Build history of the part. All positions in model axes, mm. A direction names the side the tool comes from. Round coordinates to 2 decimals unless told otherwise and drop trailing zeros. Write each loop counter-clockwise with the first axis right and the second up, starting at its lowest first coordinate (ties: lowest second). Pieces come first, ordered by that corner, then holes.
1) Saw through at D-D (x = -37.5). Write the cut outline in (y, z), plus the area to 3 significant figures.
2) Saw through at B-B (z = 109). Write the cut outline in (x, y).
3) Pull direction Y, two halves, no side cores. Call faces 6 (the flat face through (-43.288, -40.614, 68.622)), 7 (the flat face through (-1, -6, 0)), 8 (the flat face through (43.543, -41.055, 68.622)), 9 (the flat face through (12.06, 25.76, 68.62)): +Y half, -Y half, draft (parallel to the pull), parting line (faces both ways), or undercut.
4) Saw through at A-A (x = 48). Write the cut outline in (y, z), plus the area to 3 significant figures.
5) Which spindle directions (+Z, -Z, +X, -X, +Y, -Y) get a long thin tool onto all of the face, cutting with end or side? Do faces 1 (the flat face through (-42, 9.586, 69)), 2 (the flat face through (46.92, -7.99, 68.62)), 3 (the flat face through (25.9, -46.5, 68.6)), 4 (the flat face through (-47.28, -7.5, 68.62)), 5 (the flat face through (42, 9.586, 69)). Say none if no direction does.
6) Saw through at C-C (y = -22.5). Write the cut outline in (x, z), plus the area to 3 significant figures.
7) Flat gauge pins, fed straight in: pin 1 (1.5 mm diameter, centred on y = -15, z = 94.5, fed in from -X); pin 2 (2 mm diameter, centred on y = -44.5, z = 84.5, fed in from -X); pin 3 (8 mm diameter, centred on x = 31.5, z = 47, fed in from -Y); pin 4 (1 mm diameter, centred on x = -28, y = -22, fed in from -Z). Where does each tip first touch, or does it go through?
8) Wall check: probe 1 along Y at (x, z) = (50.5, 105); probe 2 along Y at (x, z) = (35.5, 83.5); probe 3 along Y at (x, z) = (19.5, 64.5). Give the ranges that are in metal, low to high.
from build123d import *

# Parameters (mm, degrees)
F1_DEPTH = 139.192
F2_R     = 27.771384
F3_DEPTH = 135.89
F5_DEPTH = 120.142


with BuildPart() as f1:
    # F0 (on Top) → F1 (new body)
    with BuildSketch(Plane.XY):
        Polygon((23.781775, 9.586452), (0, 42.401612), (-23.781775, 9.586452), (-59.915323, 9.586452), (-34.290001, -25.072258), (-52.541129, -56.596935), (0, -36.686614), (52.541129, -56.596935), (34.290001, -25.072258), (59.915323, 9.586452), align=None)
    extrude(amount=F1_DEPTH)

    # F2 (on face) → F3 (join)
    with BuildSketch(Plane(origin=(0, 0, 0), x_dir=(1, 0, 0), z_dir=(0, 0, -1))):
        with Locations((0, 6.819746)):
            Circle(F2_R)
    extrude(amount=-F3_DEPTH)

    # F4 (on face) → F5 (join)
    with BuildSketch(Plane(origin=(0, 0, 0), x_dir=(1, 0, 0), z_dir=(0, 0, -1))):
        Polygon((-13.642258, -6.452419), (0, -28.943708), (18.066773, -6.452419), (50.69758, -4.424516), (28.574999, 29.128065), (43.692097, 48.300967), (-4.793226, 31.155968), (-41.664194, 49.407098), (-27.837582, 18.619839), (-49.775805, -6.452419), align=None)
    extrude(amount=-F5_DEPTH)


solid = f1.part
Evaluation:
1. outline: (-50.9, 0) - (-30.62, 0) - (-30.62, 139.19) - (-50.9, 139.19) - close; (-20.73, 0) - (9.59, 0) - (9.59, 139.19) - (-20.73, 139.19) - close
1. area: 7,040 mm2
2. outline: (-59.92, 9.59) - (-34.29, -25.07) - (-52.54, -56.6) - (0, -36.69) - (52.54, -56.6) - (34.29, -25.07) - (59.92, 9.59) - (23.78, 9.59) - (0, 42.4) - (-23.78, 9.59) - close
3. face 6: undercut
3. face 7: draft
3. face 8: undercut
3. face 9: +Y half
4. outline: (-54.88, 0) - (-48.75, 0) - (-48.75, 139.19) - (-54.88, 139.19) - close; (-6.53, 0) - (9.59, 0) - (9.59, 139.19) - (-6.53, 139.19) - close
4. area: 3,100 mm2
5. face 1: +Z, -Z, -X, +Y
5. face 2: +Z, -Z, +X
5. face 3: +Z, -Z, -Y
5. face 4: +Z, -Z, -X
5. face 5: +Z, -Z, +X, +Y
6. outline: (-36.19, 0) - (36.19, 0) - (36.19, 139.19) - (-36.19, 139.19) - close
6. area: 10,100 mm2
7. pin 1: stops at x = -42.29
7. pin 2: stops at x = -46.12
7. pin 3: stops at y = -50.14
7. pin 4: stops at z = 0
8. probe 1: y = -55.82 to -53.07, -3.15 to 9.59
8. probe 2: y = -50.14 to -27.16, -23.44 to 9.59
8. probe 3: y = -44.08 to 15.49
